The drawing under review shows one solid part. Ordinate dimensions are in mm from its lowest x, y, z. Coordinates: 2 decimals unless noted, no trailing zeros. Write each loop counter-clockwise with the first axis right and the second up, starting at its lowest first coordinate (ties: lowest second). Pieces come first, ordered by that corner, then holes.
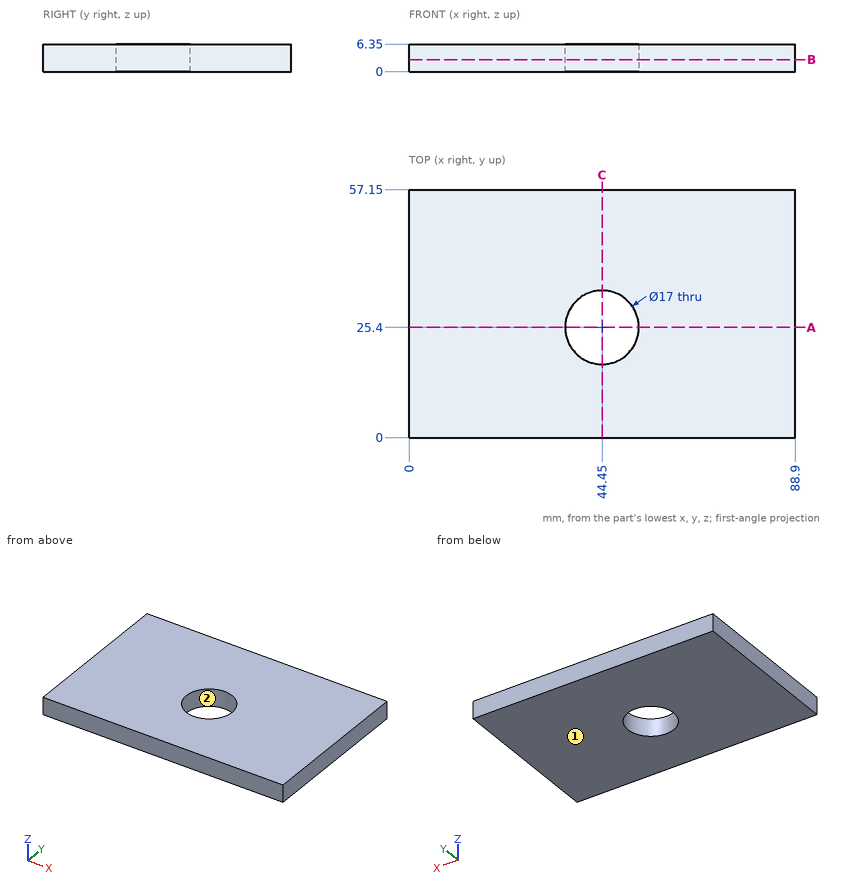
1) Consider section C-C (x = 44.45). Give the boundary of the cut face in (y, z), then the cut area to 3 significant figures.
2) Consider section A-A (y = 25.4). Give the boundary of the cut face in (x, z).
3) For L1, parallel to Y at x = 44.45, z = 4.5; L2, parallel to X at y = 21, z = 5.5; L3, parallel to Y at x = 51.5, z = 4.25, list the stretches that pass through material, from the lowest coordinate up.
4) Consider section B-B (z = 2.75). Give the boundary of the cut face in (x, y).
5) The part is to be moulded in two halves that separate along X. For the marked faces 1 and 2, say which applies: pulls with the +X half, pulls with the -X half, needs draft (parallel to the pull), parting line crosses it, or undercut.
Results:
1. outline: (0, 0) - (16.9, 0) - (16.9, 6.35) - (0, 6.35) - close; (33.9, 0) - (57.15, 0) - (57.15, 6.35) - (33.9, 6.35) - close
1. area: 255 mm2
2. outline: (0, 0) - (35.95, 0) - (35.95, 6.35) - (0, 6.35) - close; (52.95, 0) - (88.9, 0) - (88.9, 6.35) - (52.95, 6.35) - close
3. L1: y = 0 to 16.9, 33.9 to 57.15
3. L2: x = 0 to 37.18, 51.72 to 88.9
3. L3: y = 0 to 20.65, 30.15 to 57.15
4. outline: (0, 0) - (88.9, 0) - (88.9, 57.15) - (0, 57.15) - close; hole circle Ø17 at (44.45, 25.4)
5. face 1: needs draft
5. face 2: undercut
